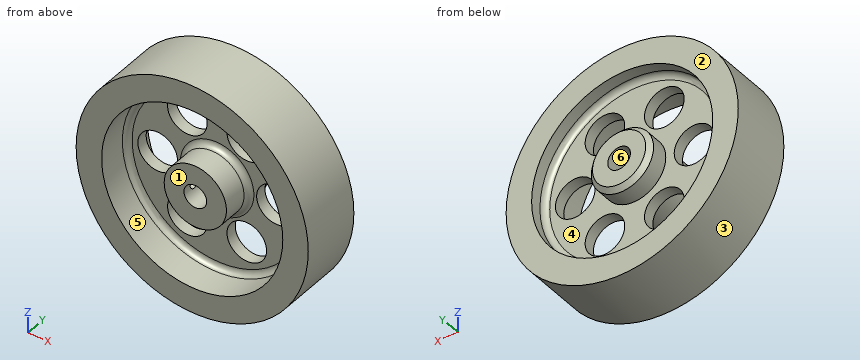
Autodesk Inventor part; units mm, degrees
ref_plane "Work Plane1" through (0, 1.5, 0) normal (0, 1, 0) x (-1, 0, 0)
ref_plane "Work Plane2" through (-11, 0, 0) normal (1, 0, 0) x (0, 1, 0)
ref_plane "XY Plane" through (0, 0, 0) normal (0, 0, 1) x (1, 0, 0)
sketch "Sketch1" plane through (0, 0, 0) normal (0, 1, 0) x (-1, 0, 0)
  circle A0 centre (0, 0) radius 41
  dimension "d0" = 82
extrude "Extrusion1" add sketch "Sketch1" along normal blind 22
sketch "Sketch2" plane through (0, 22, 0) normal (0, 1, 0) x (1, 0, 0)
  circle A0 centre (0, 0) radius 32
  dimension "d3" = 64
extrude "Extrusion2" cut sketch "Sketch2" against normal blind 6
sketch "Sketch3" plane through (0, 0, 0) normal (0, -1, 0) x (1, 0, 0)
  circle A0 centre (0, 0) radius 32
  dimension "d6" = 64
extrude "Extrusion3" cut sketch "Sketch3" against normal blind 12
ref_plane "Work Plane1" through (0, 1.5, 0) normal (0, 1, 0) x (-1, 0, 0)
sketch "Sketch4" plane through (0, 1.5, 0) normal (0, 1, 0) x (-1, 0, 0)
  circle A0 centre (0, 0) radius 11
  dimension "d10" = 22
extrude "Extrusion4" add sketch "Sketch4" along normal blind 22
sketch "Sketch5" plane through (0, 23.5, 0) normal (0, 1, 0) x (1, 0, 0)
  circle A0 centre (0, 0) radius 4
  dimension "d13" = 8
extrude "Extrusion5" cut sketch "Sketch5" against normal through all
ref_plane "Work Plane2" through (-11, 0, 0) normal (1, 0, 0) x (0, 1, 0)
sketch "Sketch6" plane through (-11, 0, 0) normal (1, 0, 0) x (0, 1, 0)
  circle A0 centre (5.9844, 0) radius 1.5
  point P0 (0, 0)
  dimension "d17" = 3
  dimension "d33" = 5.9844
extrude "Extrusion6" cut sketch "Sketch6" along normal blind 10
sketch "Sketch7" plane through (0, 12, 0) normal (0, -1, 0) x (1, 0, 0)
  circle A0 centre (20.9744, 0) radius 7
  circle A1 centre (10.4872, 18.1643) radius 7
  circle A2 centre (-10.4872, 18.1643) radius 7
  circle A3 centre (-20.9744, 0) radius 7
  circle A4 centre (-10.4872, -18.1643) radius 7
  circle A5 centre (10.4872, -18.1643) radius 7
  point P0 (0, 0)
  dimension "d20" = 14
  dimension "d23" = 360
  dimension "d34" = 20.9744
extrude "Extrusion7" cut sketch "Sketch7" against normal through all
fillet "Fillet1" radius 2 1 edges at (11, 12, 0)
fillet "Fillet2" radius 2 1 edges at (-32, 12, 0)
fillet "Fillet3" radius 2 1 edges at (-32, 16, 0)
chamfer "Chamfer1" distance 1.6 angle 45 1 edges at (11, 23.5, 0)
properties part number "reverse gear fly wheel"
Source: CAD feature listing. Evaluate the final solid. Frame: model axes, mm. Face numbers are marked on the shaded views. A direction names the side the tool comes from. Give positions to 0.01 mm unless a question says otherwise; leave off trailing zeros. Write each loop counter-clockwise with the first axis right and the second up, starting at its lowest first coordinate (ties: lowest second). Pieces come first, ordered by that corner, then holes. Notation, with made-up numbers: M -28,-21.5 L 12,-21.5 A30 ccw 12,14.5 Z; hole C -23.5,75 d10. An arc over 180 degrees is marked long. Return JSON: item names as keys, results as strings. Group by question number.
1) Set-up query: the marked faces 4, 5 and 6. Return all of +Z, -Z, +X, -X, +Y, -Y with unobstructed straight access to the full face (end or side cutting, diameter ignored); none if empty.
2) Cut plane D-D, the plane z = 0. Give the number of separate pieces and of enclosed holes in the cut face, plus the area to 3 significant figures.
3) Pin query (flat end, axial travel): P1, Ø8.5, axis at x = -10.49, z = -18.16, coming from the +Y side; P2, Ø3, axis at y = 14.5, z = 19, coming from the +X side; P3, Ø12, axis at x = 18.5, y = 13.5, coming from the -Z side; P4, Ø8, axis at y = 3.5, z = -22.5, coming from the +X side. Return the tip coordinate at first contact, or that it passes through.
4) Pull-direction query (Z, two-part tool) for the marked faces 1, 2 and 3; classes: pulls with the +Z half, pulls with the -Z half, needs draft (parallel to the pull), parting line crosses it, or undercut.
5) Cut plane C-C, the plane y = 14.5. Output: boundary loops of the cut face in (x, z).
6) Material intervals for line 1 along Z through (x, y) = (0, 21.2); line 2 along X through (y, z) = (17.5, -6.5); line 3 along Z through (x, y) = (8.5, 6.5), sorted ascending. Write a range as [from, to].
7) Cut plane B-B, the plane y = 3. Output: boundary loops of the cut face in (x, z).
Recorded:
{
 "1": {"face 4": "+Y", "face 5": "-Y", "face 6": "+Y, -Y"},
 "2": {"separate pieces": "5", "enclosed holes": "0", "area": "742 mm²"},
 "3": {"P1": "passes through", "P2": "stops at x = 37.08", "P3": "stops at z = -39.05", "P4": "stops at x = 36.59"},
 "4": {"face 1": "undercut", "face 2": "needs draft", "face 3": "parting line crosses it"},
 "5": {"outline": "C 0,0 d82; hole C -20.97,0 d14; hole C -10.49,-18.16 d14; hole C -10.49,18.16 d14; hole C 0,0 d8; hole C 10.49,-18.16 d14; hole C 10.49,18.16 d14; hole C 20.97,0 d14"},
 "6": {"line 1": "z = [-41, -32], [-11, -4], [4, 11], [32, 41]", "line 2": "x = [-40.48, -31.27], [-8.87, 8.87], [31.27, 40.48]", "line 3": "z = [-40.11, -30.85], [-6.98, 6.98], [30.85, 40.11]"},
 "7": {"outline": "C 0,0 d82; C 0,0 d22; hole C 0,0 d64; hole C 0,0 d8"}
}
